Source: CAD feature listing. Evaluate the final solid. Frame: model axes, mm. A direction names the side the tool comes from. Give positions to 0.01 mm unless a question says otherwise; leave off trailing zeros. Loops run counter-clockwise (first coordinate to the right, second up) from the corner with the lowest first, then second, coordinate; pieces in that order, holes last.
```python
from build123d import *

# Parameters (mm, degrees)
SKETCH1_W           = 177.8
SKETCH1_H           = 254
BOSS_EXTRUDE1_DEPTH = 36.445
SHELL1_T            = 3
SKETCH2_R           = 22
SKETCH2_R_2         = 2.5
CUT_EXTRUDE1_DEPTH  = 3
SKETCH3_R           = 5
CUT_EXTRUDE2_DEPTH  = 3
SKETCH12_W          = 12
SKETCH12_H          = 66.89
BOSS_EXTRUDE5_DEPTH = 8
SKETCH10_R          = 3
CUT_EXTRUDE8_DEPTH  = 8
SKETCH13_W          = 174.8
SKETCH13_H          = 69.89
SKETCH13_W_2        = 171.8
SKETCH13_H_2        = 66.89
BOSS_EXTRUDE6_DEPTH = 25
SKETCH14_W          = 175.3
SKETCH14_H          = 70.39
SKETCH14_W_2        = 171.8
SKETCH14_H_2        = 66.89
CUT_EXTRUDE9_DEPTH  = 10
SKETCH17_W          = 171.8
SKETCH17_H          = 66.89
BOSS_EXTRUDE7_DEPTH = 2
SKETCH22_W          = 5
SKETCH22_H          = 5
CUT_EXTRUDE14_DEPTH = 5
BOSS_EXTRUDE8_DEPTH = 5
CUT_EXTRUDE12_DEPTH = 5
SKETCH21_W          = 23.209480822
SKETCH21_H          = 1.5
CUT_EXTRUDE13_DEPTH = 5


with BuildPart() as part:
    # Sketch1 → Boss-Extrude1 (new, symmetric)
    with BuildSketch(Plane.XY):
        Rectangle(SKETCH1_W, SKETCH1_H)
    extrude(amount=BOSS_EXTRUDE1_DEPTH, both=True)

    # Shell1 (no face opened: a closed hollow body)
    add(offset(amount=-SHELL1_T, mode=Mode.PRIVATE), mode=Mode.SUBTRACT)

    # Sketch2 → Cut-Extrude1 (cut)
    with BuildSketch(Plane(origin=(0, 0, 33.445), x_dir=(-1, 0, 0), z_dir=(0, 0, -1))):
        with Locations((0, -4)):
            Circle(SKETCH2_R)
        with Locations((-3.75, -47.907937278)):
            Circle(SKETCH2_R_2)
        with Locations((3.75, -47.907937278)):
            Circle(SKETCH2_R_2)
        with Locations((-57.788969133, -0.25)):
            Circle(SKETCH2_R_2)
        with Locations((-57.788969133, -7.75)):
            Circle(SKETCH2_R_2)
        with Locations(Location((57.788969133, -0.25, 0), (0, 0, 180))):
            Circle(SKETCH2_R_2)
        with Locations(Location((57.788969133, -7.75, 0), (0, 0, 180))):
            Circle(SKETCH2_R_2)
        with Locations(Location((3.75, 39.907937278, 0), (0, 0, 180))):
            Circle(SKETCH2_R_2)
        with Locations(Location((-3.75, 39.907937278, 0), (0, 0, 180))):
            Circle(SKETCH2_R_2)
    extrude(amount=-CUT_EXTRUDE1_DEPTH, mode=Mode.SUBTRACT)

    # Sketch3 → Cut-Extrude2 (cut)
    with BuildSketch(Plane.XY.offset(-33.445)):
        with Locations((-20.9, 34)):
            Circle(SKETCH3_R)
    extrude(amount=-CUT_EXTRUDE2_DEPTH, mode=Mode.SUBTRACT)

    # Sketch12 → Boss-Extrude5 (add)
    with BuildSketch(Plane.XZ.offset(-124)):
        Rectangle(SKETCH12_W, SKETCH12_H)
    extrude(amount=BOSS_EXTRUDE5_DEPTH)

    # Sketch10 → Cut-Extrude8 (cut)
    with BuildSketch(Plane(origin=(0, 127, 0), x_dir=(1, 0, 0), z_dir=(0, 1, 0))):
        with Locations(Location((0, 0, 0), (0, 0, 270))):
            Circle(SKETCH10_R)
    extrude(amount=-CUT_EXTRUDE8_DEPTH, mode=Mode.SUBTRACT)


with BuildPart() as body_2:
    # Split2: the piece on the far side of the plane
    add(part.part)
    split(bisect_by=Plane.ZX.offset(52), keep=Keep.BOTTOM)

    # Sketch13 → Boss-Extrude6 (add)
    with BuildSketch(Plane(origin=(0, 52, 0), x_dir=(1, 0, 0), z_dir=(0, 1, 0))):
        Rectangle(SKETCH13_W, SKETCH13_H)
        Rectangle(SKETCH13_W_2, SKETCH13_H_2, mode=Mode.SUBTRACT)
    extrude(amount=BOSS_EXTRUDE6_DEPTH)

    # Sketch17 → Boss-Extrude7 (add)
    with BuildSketch(Plane(origin=(0, -124, 0), x_dir=(1, 0, 0), z_dir=(0, 1, 0))):
        Rectangle(SKETCH17_W, SKETCH17_H)
    extrude(amount=BOSS_EXTRUDE7_DEPTH)

    # Sketch22 → Cut-Extrude14 (cut)
    with BuildSketch(Plane.XZ.offset(127)):
        Polygon((11.604740411, 0), (5.802370205, 10.05), (-5.802370205, 10.05), (-11.604740411, 0), (-5.802370205, -10.05), (5.802370205, -10.05), align=None)
        with Locations((-17.67766953, 17.67766953)):
            Rectangle(SKETCH22_W, SKETCH22_H)
        with Locations((17.67766953, 17.67766953)):
            Rectangle(SKETCH22_W, SKETCH22_H)
        with Locations((17.67766953, -17.67766953)):
            Rectangle(SKETCH22_W, SKETCH22_H)
        with Locations((-17.67766953, -17.67766953)):
            Rectangle(SKETCH22_W, SKETCH22_H)
    extrude(amount=-CUT_EXTRUDE14_DEPTH, mode=Mode.SUBTRACT)


with BuildPart() as part_1:
    add(part.part)

    # Split2
    split(bisect_by=Plane.ZX.offset(52), keep=Keep.TOP)

    # Sketch14 → Cut-Extrude9 (cut)
    with BuildSketch(Plane.XZ.offset(-52)):
        Rectangle(SKETCH14_W, SKETCH14_H)
        Rectangle(SKETCH14_W_2, SKETCH14_H_2, mode=Mode.SUBTRACT)
    extrude(amount=-CUT_EXTRUDE9_DEPTH, mode=Mode.SUBTRACT)


with BuildPart() as body_3:
    # Split3: the piece on the far side of the plane
    add(body_2.part)
    split(bisect_by=Plane.XY, keep=Keep.BOTTOM)

    # Sketch19 → Boss-Extrude8 (add)
    with BuildSketch(Plane.XY):
        Polygon((-87.4, 77), (-85.9, 77), (-85.9, 75.5), (-85.9, -122), (-11.604740411, -122), (-11.604740411, -123.5), (-87.4, -123.5), align=None)
        Polygon((87.4, 77), (87.4, -123.5), (11.604740411, -123.5), (11.604740411, -122), (85.9, -122), (85.9, 75.5), (85.9, 77), align=None)
    extrude(amount=BOSS_EXTRUDE8_DEPTH)


with BuildPart() as body_2_1:
    add(body_2.part)

    # Split3
    split(bisect_by=Plane.XY, keep=Keep.TOP)

    # Sketch20 → Cut-Extrude12 (cut)
    with BuildSketch(Plane(origin=(0, 0, 0), x_dir=(-1, 0, 0), z_dir=(0, 0, -1))):
        Polygon((-87.4, 77), (-87.4, -123.5), (-11.604740411, -123.5), (-11.604740411, -122), (-85.9, -122), (-85.9, 77), align=None)
        Polygon((85.9, 77), (85.9, -122), (11.604740411, -122), (11.604740411, -123.5), (87.4, -123.5), (87.4, 77), align=None)
    extrude(amount=-CUT_EXTRUDE12_DEPTH, mode=Mode.SUBTRACT)

    # Sketch21 → Cut-Extrude13 (cut)
    with BuildSketch(Plane(origin=(0, 0, 0), x_dir=(-1, 0, 0), z_dir=(0, 0, -1))):
        with Locations((0, -122.75)):
            Rectangle(SKETCH21_W, SKETCH21_H)
    extrude(amount=-CUT_EXTRUDE13_DEPTH, mode=Mode.SUBTRACT)


solid = body_2_1.part
```
(1) Section C-C, the plane x = -50.5. Return the cut outline in (y, z) (3 decimals).
A:
outline: (-127, 0) - (-123.5, 0) - (-123.5, 5) - (-122, 5) - (-122, 33.445) - (77, 33.445) - (77, 34.945) - (52, 34.945) - (52, 36.445) - (-127, 36.445) - close
(2) Mould query, pull axis Z, two halves, no side actions, for faces 1 (the flat face through (20.178, -125, 18)), 2 (the flat face through (-1, -127, 18)), 3 (the flat face through (8.744, -125.091, 4.955)). Classes: pulls with the +Z half, pulls with the -Z half, needs draft (parallel to the pull), parting line crosses it, or undercut.
A:
face 1: undercut
face 2: needs draft
face 3: pulls with the -Z half
(3) Section B-B, the plane z = 29. Return the cut outline in (x, y), then the cut area to 3 significant figures.
A:
outline: (-88.9, -127) - (88.9, -127) - (88.9, 52) - (87.4, 52) - (87.4, 77) - (85.9, 77) - (85.9, -122) - (-85.9, -122) - (-85.9, 77) - (-87.4, 77) - (-87.4, 52) - (-88.9, 52) - close
area: 2,010 mm2
(4) Ray query, line 1 along Y through (x, z) = (0, 35); line 2 along X through (y, z) = (19, 20.5); line 3 along Y through (x, z) = (3.75, 34.6). Return the intervals inside material, ascending.
A:
line 1: y = -127 to -26, 18 to 52
line 2: x = -88.9 to -85.9, 85.9 to 88.9
line 3: y = -127 to -50.41, -45.41 to -25.68, 17.68 to 37.41, 42.41 to 77
(5) Section A-A, the plane y = -21. Return the cut outline in (x, z) (3 decimals).
A:
outline: (-88.9, 0) - (-87.4, 0) - (-87.4, 5) - (-85.9, 5) - (-85.9, 33.445) - (-13.964, 33.445) - (-13.964, 36.445) - (-88.9, 36.445) - close; (13.964, 33.445) - (85.9, 33.445) - (85.9, 5) - (87.4, 5) - (87.4, 0) - (88.9, 0) - (88.9, 36.445) - (13.964, 36.445) - close
(6) First-contact query: pin 1 (14 mm diameter, centred on x = 37, z = 20.5, fed in from +Y); pin 2 (4 mm diameter, centred on x = -57.79, y = -0.25, fed in from +Z); pin 3 (6 mm diameter, centred on x = -57.79, y = -7.75, fed in from -Z) (3 decimals). Flat tips, straight axial feed; report the tip coordinate or a pass-through.
A:
pin 1: stops at y = -122
pin 2: passes through
pin 3: stops at z = 33.445
(7) Reachability of faces 4 (the flat face through (-8.66, -125.09, 5.1)), 5 (the flat face through (87.4, 64, 20)), 6 (the flat face through (-18, -125, 20.178)), 7 (the flat face through (-1, 64, 34.945)) from +Z, -Z, +X, -X, +Y, -Y: full face, straight path, thin tool, end or side. Return the list, or none.
A:
face 4: -Z, +Y, -Y
face 5: +Z, -Z, +X, +Y
face 6: +Y, -Y
face 7: +Z, +X, -X, +Y
(8) Section D-D, the plane y = -79. Return the cut outline in (x, z) (3 decimals).
A:
outline: (-88.9, 0) - (-87.4, 0) - (-87.4, 5) - (-85.9, 5) - (-85.9, 33.445) - (85.9, 33.445) - (85.9, 5) - (87.4, 5) - (87.4, 0) - (88.9, 0) - (88.9, 36.445) - (-88.9, 36.445) - close
